Autodesk Fusion 360 part; units mm, degrees
sketch "Skizze1" plane through (0, 0, 0) normal (1, 0, 0) x (0, 0, -1)
  circle A0 centre (0, 0) radius 3
  circle A1 centre (0, 0) radius 2
  dimension "d1" = 6
  dimension "d2" = 4
extrude "Extrusion1" add sketch "Skizze1" along normal blind 40 makes body 1
copy_body "Körper->Berechn1" bodies 1 removing the originals makes body 2 in component "SwagelokTube"
component "SwagelokTube" placed x (1, 0, 0) y (0, 1, 0) z (0, 0, 1) at (0, 0, 0)
Read the model definition and answer for the solid it produces. Units are mm, in the model's axes. Coordinates: 2 decimals unless noted, no trailing zeros. Write each loop counter-clockwise with the first axis right and the second up, starting at its lowest first coordinate (ties: lowest second). Pieces come first, ordered by that corner, then holes. Notation, with made-up numbers: (-16.5, 25.25) -> (40.5, 25.25) arc R24 cw to (40.5, 53.25) -> close; hole circle Ø8 at (-2.75, 54). An arc over 180 degrees is marked (long way). Answer as a JSON object with one key per item and string values.
Q1. Flat-ended cylindrical pins translate along their axes: pin 1 Ø3 at (y, z) = (0, 0) entering from -X; pin 2 Ø1 at (x, y) = (18, -1) entering from +Z. Find the tip coordinate at first contact, or state that the pin passes through.
The answers:
{"pin 1": "passes through", "pin 2": "stops at z = 2.96"}
Q2. Determine the mould class of faces 1 (the flat face through (0, -2, -1)), 2 (the cylindrical face through (20, 0, 3)), 3 (the cylindrical face through (20, 2, 0)) for opening direction Z: pulls with the +Z half, pulls with the -Z half, needs draft (parallel to the pull), parting line crosses it, or undercut.
The answers:
{"face 1": "needs draft", "face 2": "parting line crosses it", "face 3": "undercut"}
Q3. Consider line 1 (Y direction, x = 13.5, z = 0); line 2 (Z direction, x = 32.5, y = -0.5); line 3 (Y direction, x = 8, z = 1.75). Determine where each line is inside the solid, lowest interval first. Write a range as [from, to].
The answers:
{"line 1": "y = [-3, -2], [2, 3]", "line 2": "z = [-2.96, -1.94], [1.94, 2.96]", "line 3": "y = [-2.44, -0.97], [0.97, 2.44]"}
Q4. The part is cut by section D-D on z = -2.45. Give the vertices of the cut face in (x, y).
The answers:
{"outline": "(0, -1.73) -> (40, -1.73) -> (40, 1.73) -> (0, 1.73) -> close"}
Q5. The part is cut by section A-A on y = 0. Give the vertices of the cut face in (x, z).
The answers:
{"outline": "(0, -3) -> (40, -3) -> (40, -2) -> (0, -2) -> close; (0, 2) -> (40, 2) -> (40, 3) -> (0, 3) -> close"}
Q6. The part is cut by section C-C on x = 30.5. Give the vertices of the cut face in (y, z), then the cut area to 3 significant figures.
The answers:
{"outline": "circle Ø6 at (0, 0); hole circle Ø4 at (0, 0)", "area": "15.7 mm2"}
